from build123d import *

# Parameters (mm, degrees)
BOSS_EXTRUDE1_DEPTH                                 = 12.7
CHAMFER1_SIZE2                                      = 47.397045256
CHAMFER1_SIZE                                       = 12.7
CSK_FOR_1_4_FLAT_HEAD_MACHINE_SCREW_100_D           = 7.14248
CSK_FOR_1_4_FLAT_HEAD_MACHINE_SCREW_100_CSINK_D     = 13.716
CSK_FOR_1_4_FLAT_HEAD_MACHINE_SCREW_100_CSINK_ANGLE = 100
LPATTERN1_COUNT                                     = 3
LPATTERN1_PITCH                                     = 381


with BuildPart() as part:
    # Sketch1 → Boss-Extrude1 (new body)
    with BuildSketch(Plane(origin=(0, 0, 0), x_dir=(1, 0, 0), z_dir=(0, 1, 0))):
        Polygon((-457.2, 0), (457.2, 0), (740.264592562, -292.1), (-457.2, -292.1), align=None)
    extrude(amount=BOSS_EXTRUDE1_DEPTH)

    # Chamfer1
    chamfer1_edges = [part.edges().sort_by_distance(p)[0] for p in [
        (141.532296281, 0, 292.1),
    ]]
    chamfer1_side = [part.faces().sort_by_distance(p)[0] for p in [
        (141.532296281, 0.254, 292.1),
    ]]
    chamfer(chamfer1_edges, length=CHAMFER1_SIZE - 0.0001, length2=CHAMFER1_SIZE2 - 0.0001, reference=chamfer1_side[0])  # a hair under: the kernel refuses the full size

    # CSK for 1/4 Flat Head Machine Screw (100)1 (through all)
    with Locations(Plane(origin=(0, 12.7, 0), x_dir=(1, 0, 0), z_dir=(0, 1, 0))):
        with Locations((-381, -44.45), (-381, -196.85)):
            csk_for_1_4_flat_head_machine_screw_100 = CounterSinkHole(CSK_FOR_1_4_FLAT_HEAD_MACHINE_SCREW_100_D / 2, CSK_FOR_1_4_FLAT_HEAD_MACHINE_SCREW_100_CSINK_D / 2, counter_sink_angle=CSK_FOR_1_4_FLAT_HEAD_MACHINE_SCREW_100_CSINK_ANGLE)

    # LPattern1: CSK for 1/4 Flat Head Machine Screw (100)1 ×3
    with Locations(*[(i * LPATTERN1_PITCH, 0, 0) for i in range(1, LPATTERN1_COUNT)]):
        add(csk_for_1_4_flat_head_machine_screw_100, mode=Mode.SUBTRACT)


solid = part.part
The listing builds one solid part. Answer for the finished solid, in the listing's coordinates (mm). Round coordinates to 2 decimals unless told otherwise and drop trailing zeros. Loops run counter-clockwise (first coordinate to the right, second up) from the corner with the lowest first, then second, coordinate; pieces in that order, holes last. Notation, with made-up numbers: M 14.5,15 L 62.5,15 A34 ccw 62.5,51 Z; hole C 5,81 d4. An arc over 180 degrees is marked long. Write each question's results on one line, items separated by ' | '. Start each with the question number.
1) Find section D-D on z = 148. Write down the section's boundary in (x, y).
2) Find section A-A on y = 4.25. Write down the section's boundary in (x, z), plus the area to 3 significant figures.
3) Each of these flat-tipped pins is pushed along its axis until it touches: pin 1 (5.5 mm diameter, centred on x = -381, z = 44.45, fed in from -Y); pin 2 (8 mm diameter, centred on x = 0, z = 196.85, fed in from +Y); pin 3 (5 mm diameter, centred on y = 2.5, z = 140, fed in from +X); pin 4 (4 mm diameter, centred on y = 7, z = 175.5, fed in from +X). Where does it stop, or does it pass through?
4) Straight lines are drawn through the part: probe 1 along X at (y, z) = (6.25, 44.45); probe 2 along X at (y, z) = (6.5, 196.85); probe 3 along Y at (x, z) = (-408, 256.5). For each, find the intervals that lie inside material, in ascending order.
5) Find section C-C on z = 72. Write down the section's boundary in (x, y).
Final values:
1) outline: M -457.2,0 L 600.62,0 L 600.62,12.7 L -457.2,12.7 Z
2) outline: M -457.2,0 L 457.2,0 L 709.7,260.56 L -457.2,260.56 Z; hole C -381,44.45 d7.14; hole C -381,196.85 d7.14; hole C 0,44.45 d7.14; hole C 0,196.85 d7.14; hole C 381,44.45 d7.14; hole C 381,196.85 d7.14 | area: 271,000 mm²
3) pin 1: through | pin 2: y = 10.3 | pin 3: x = 595.29 | pin 4: x = 629.21
4) probe 1: -457.2 to -384.57, -377.43 to -3.57, 3.57 to 377.43, 384.57 to 500.28 | probe 2: -457.2 to -384.57, -377.43 to -3.57, 3.57 to 377.43, 384.57 to 647.96 | probe 3: 3.16 to 12.7
5) outline: M -457.2,0 L 526.97,0 L 526.97,12.7 L -457.2,12.7 Z
